from build123d import *

# Parameters (mm, degrees)
BOSS_EXTRUDE1_DEPTH = 76.2
SKETCH4_R           = 2.54
CUT_EXTRUDE2_DEPTH  = 76.2


with BuildPart() as part:
    # Sketch1 → Boss-Extrude1 (new body)
    with BuildSketch(Plane.XY):
        with BuildLine():
            Line((0, 5.08), (0, 76.2))
            Line((0, 76.2), (12.7, 76.2))
            Line((12.7, 76.2), (12.7, 17.78))
            ThreePointArc((12.7, 17.78), (14.187897552, 14.187897552), (17.78, 12.7))
            Line((17.78, 12.7), (127, 12.7))
            Line((127, 12.7), (127, 0))
            Line((127, 0), (5.08, 0))
            ThreePointArc((5.08, 0), (1.487897552, 1.487897552), (0, 5.08))
        make_face()
    extrude(amount=BOSS_EXTRUDE1_DEPTH)

    # Sketch4 → Cut-Extrude2 (cut)
    with BuildSketch(Plane.ZY):
        with Locations((9.284401907, 67.53455822)):
            Circle(SKETCH4_R)
        with Locations((66.915598093, 67.53455822)):
            Circle(SKETCH4_R)
        with Locations((66.915598093, 25.4)):
            Circle(SKETCH4_R)
        with Locations((9.284401907, 25.4)):
            Circle(SKETCH4_R)
    extrude(amount=-CUT_EXTRUDE2_DEPTH, mode=Mode.SUBTRACT)


solid = part.part
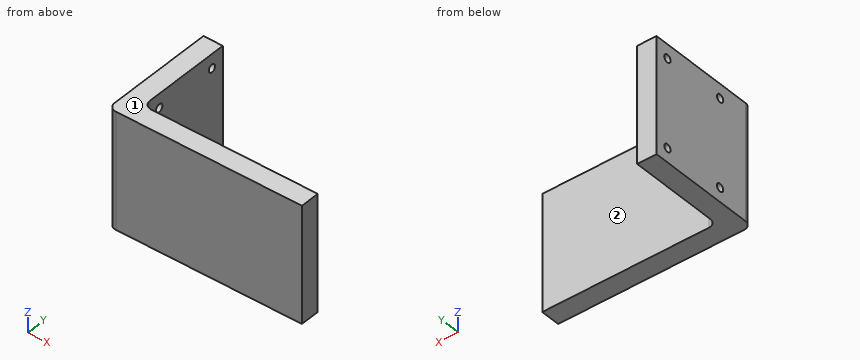
Verification items for the finished model (mm, model axes). Face numbers are marked on the shaded views. A direction names the side the tool comes from. Coordinates: 2 decimals unless noted, no trailing zeros. Order: outer loops, then holes, each group sorted by start corner. A loop starts at its lowest first (then second) coordinate and runs counter-clockwise, first axis right, second up.
Item 1: Section check B-B, the plane z = 22. Enter the section's corners in (x, y).
Filled in:
outline: (0, 5.08) arc R5.08 ccw to (5.08, 0) - (127, 0) - (127, 12.7) - (17.78, 12.7) arc R5.08 cw to (12.7, 17.78) - (12.7, 76.2) - (0, 76.2) - close
Item 2: Access from +Z, -Z, +X, -X, +Y, -Y to the whole of each face (thin tool, end or side, straight path). Record for the marked faces 1 and 2.
Filled in:
face 1: +Z, +X, -X, +Y, -Y
face 2: +Z, -Z, +X, +Y
Item 3: Section check C-C, the plane x = 119. Enter the section's corners in (y, z), then the cut area to 3 significant figures.
Filled in:
outline: (0, 0) - (12.7, 0) - (12.7, 76.2) - (0, 76.2) - close
area: 968 mm2
Item 4: Material ranges on L1, parallel to Y at x = 51, z = 14.5; L2, parallel to X at y = 16, z = 12.5, recorded low to high.
Filled in:
L1: y = 0 to 12.7
L2: x = 0 to 13.02
Item 5: Section check A-A, the plane y = 25.4. Enter the section's corners in (x, z), then the cut area to 3 significant figures.
Filled in:
outline: (0, 0) - (12.7, 0) - (12.7, 6.74) - (0, 6.74) - close; (0, 11.82) - (12.7, 11.82) - (12.7, 64.38) - (0, 64.38) - close; (0, 69.46) - (12.7, 69.46) - (12.7, 76.2) - (0, 76.2) - close
area: 839 mm2
Item 6: Depth check by flat-ended pin: pin 1 (2 mm diameter, centred on y = 63, z = 32.5, fed in from +X); pin 2 (10 mm diameter, centred on x = 43, z = 24.5, fed in from +Y); pin 3 (1 mm diameter, centred on y = 51, z = 24.5, fed in from -X). Enter the tip coordinate at first touch or a pass-through.
Filled in:
pin 1: stops at x = 12.7
pin 2: stops at y = 12.7
pin 3: stops at x = 0
